Work out the finished part from the listing and answer in its coordinate system (mm). A direction names the side the tool comes from. Coordinates: 2 decimals unless noted, no trailing zeros. Order: outer loops, then holes, each group sorted by start corner. A loop starts at its lowest first (then second) coordinate and runs counter-clockwise, first axis right, second up.
1. The part is cut by section D-D, the plane z = -31.5. Give the vertices of the cut face in (x, y).
2. Flat-ended cylindrical pins translate along their axes: pin 1 Ø3 at (y, z) = (1.5, -36.5) entering from +X; pin 2 Ø5 at (y, z) = (5.5, -27.5) entering from -X; pin 3 Ø1.2 at (x, y) = (2.5, 4) entering from +Z. Find the tip coordinate at first contact, or state that the pin passes through.
3. A tool of negligible diameter and unlimited length cuts with its end or side. For faces 4 (the flat face through (2, 5, -103)), 5 (the flat face through (-93.68, 1.43, 51.74)), 6 (the flat face through (-101, 5, 8.672)), 7 (the flat face through (-92, 2.9, 51)), from which of +Z, -Z, +X, -X, +Y, -Y can it reach the whole face along a straight path? Write none if from no direction.
4. Determine the mould class of faces 1 (the flat face through (-4, 5, -105)), 2 (the flat face through (2, 7, -105)), 3 (the flat face through (-43, 7, -92)) for opening direction Y: +Y half, -Y half, draft (parallel to the pull), parting line (faces both ways), or undercut.
5. The part is cut by section A-A, the plane z = 12. Give the vertices of the cut face in (x, y).
6. The part is cut by section C-C, the plane x = -81. Give the vertices of the cut face in (y, z), then the cut area to 3 significant figures.
7. The part is cut by section B-B, the plane y = 5. Count the separate pieces of the cut face and the enclosed holes in it, then the cut area to 3 significant figures.
8. Find the intervals of material crossed by probe 1 along Z at (x, y) = (-91.5, 0.5); probe 2 along Z at (x, y) = (-2, 4.75); probe 3 along X at (y, z) = (3.5, 27.5), in increasing order.
```python
from build123d import *

# Parameters (mm, degrees)
BOSS_EXTRUDE1_DEPTH             = 10
SKETCH2_W                       = 8
SKETCH2_H                       = 4.2
CUT_EXTRUDE1_DEPTH              = 4
SKETCH3_W                       = 8
SKETCH3_H                       = 4
BOSS_EXTRUDE2_DEPTH             = 4
SKETCH4_W                       = 8
SKETCH4_H                       = 4
CUT_EXTRUDE2_DEPTH              = 104
CIRPATTERN4_COUNT               = 5
CIRPATTERN4_ANGLE               = 72
CIRPATTERN4_THE_OTHER_WAY_COUNT = 5
CIRPATTERN4_THE_OTHER_WAY_ANGLE = 72


with BuildPart() as part:
    # Sketch1 → Boss-Extrude1 (new body)
    with BuildSketch(Plane(origin=(0, 0, 0), x_dir=(1, 0, 0), z_dir=(0, 1, 0))):
        with BuildLine():
            Line((-4, 107), (-4, 102.92230079))
            ThreePointArc((-4, 102.92230079), (-89.20061659, 51.5), (-91.1333271, -47.99704878))
            Line((-91.1333271, -47.99704878), (-94.664718205, -50.035898385))
            Line((-94.664718205, -50.035898385), (-92.664718205, -53.5))
            Line((-92.664718205, -53.5), (-86.602540378, -50))
            ThreePointArc((-86.602540378, -50), (-86.602540378, 50), (0, 100))
            Line((0, 100), (0, 107))
            Line((0, 107), (-4, 107))
        make_face()
    extrude(amount=BOSS_EXTRUDE1_DEPTH)

    # Sketch2 → Cut-Extrude1 (cut)
    with BuildSketch(Plane(origin=(-92.664718205, 0, 53.5), x_dir=(0.5, 0, 0.866025404), z_dir=(-0.866025404, 0, 0.5))):
        with Locations((0, 5)):
            Rectangle(SKETCH2_W, SKETCH2_H)
    extrude(amount=-CUT_EXTRUDE1_DEPTH, mode=Mode.SUBTRACT)

    # Sketch3 → Boss-Extrude2 (add)
    with BuildSketch(Plane(origin=(0, 0, -107), x_dir=(-1, 0, 0), z_dir=(0, 0, -1))):
        with Locations((0, 5)):
            Rectangle(SKETCH3_W, SKETCH3_H)
    extrude(amount=-BOSS_EXTRUDE2_DEPTH)

    # Sketch4 → Cut-Extrude2 (cut, through all)
    with BuildSketch(Plane(origin=(0, 0, 0), x_dir=(0, 0, -1), z_dir=(1, 0, 0))):
        with Locations((-12.672320837, 5)):
            Rectangle(SKETCH4_W, SKETCH4_H)
    cut_extrude2 = extrude(amount=-CUT_EXTRUDE2_DEPTH, mode=Mode.SUBTRACT)

    # CirPattern4: Cut-Extrude2 ×5 about axis
    cirpattern4_axis = Axis((0, 0, 0), (0, -1, 0))
    for i in range(1, CIRPATTERN4_COUNT):
        add(cut_extrude2.rotate(cirpattern4_axis, i * CIRPATTERN4_ANGLE / (CIRPATTERN4_COUNT - 1)), mode=Mode.SUBTRACT)

    # CirPattern4 the other way: Cut-Extrude2 ×5 about axis
    cirpattern4_the_other_way_axis = Axis((0, 0, 0), (0, 1, 0))
    for i in range(1, CIRPATTERN4_THE_OTHER_WAY_COUNT):
        add(cut_extrude2.rotate(cirpattern4_the_other_way_axis, i * CIRPATTERN4_THE_OTHER_WAY_ANGLE / (CIRPATTERN4_THE_OTHER_WAY_COUNT - 1)), mode=Mode.SUBTRACT)


solid = part.part
```
Geometry says:
1. outline: (-98.07, 0) - (-94.91, 0) - (-94.91, 10) - (-98.07, 10) - close
2. pin 1: stops at x = -92.5
2. pin 2: stops at x = -99.92
2. pin 3: stops at z = -103
3. face 4: +Z, +X, +Y, -Y
3. face 5: +Z, -X, +Y, -Y
3. face 6: +X, -X
3. face 7: +Z, -X
4. face 1: draft
4. face 2: +Y half
4. face 3: undercut
5. outline: (-102.3, 0) - (-99.28, 0) - (-99.28, 3) - (-102.3, 3) - close; (-102.3, 7) - (-99.28, 7) - (-99.28, 10) - (-102.3, 10) - close
6. outline: (0, -63.62) - (10, -63.62) - (10, -58.64) - (0, -58.64) - close
6. area: 49.8 mm2
7. separate pieces: 7
7. enclosed holes: 0
7. area: 525 mm2
8. probe 1: z = -47.29 to -40.35, 40.35 to 47.29, 48.21 to 52.83
8. probe 2: z = -107 to -99.98
8. probe 3: x = -99.26 to -96.14
